Design review of the part shown in the three views and the two pictorial views. Dimensions are in mm from the part's minimum x, y and z. A direction names the side the tool comes from. Round coordinates to 2 decimals unless told otherwise and drop trailing zeros. Loops run counter-clockwise (first coordinate to the right, second up) from the corner with the lowest first, then second, coordinate; pieces in that order, holes last.
1) Take a section at B-B (y = 37.5). State the section outline as (x, z) points (3 decimals), then the cut area to 3 significant figures.
2) Take a section at D-D (y = 10.5). State the section outline as (x, z) points, then the cut area to 3 significant figures.
3) Insertion check: pin 1 (7.5 mm diameter, centred on x = 4, z = 17, fed in from -Y); pin 2 (4.5 mm diameter, centred on x = 7.5, y = 37.5, fed in from -Z); pin 3 (7.5 mm diameter, centred on x = 4.5, z = 15, fed in from +Y); pin 4 (2 mm diameter, centred on y = 16.5, z = 5, fed in from +X). Each pin has a flat end and moves straight along its axis. Give the tip position at first contact, or say it passes through.
4) Wall thickness on L1, parallel to X at y = 37.5, z = 37.95 (3 decimals); L2, parallel to Y at x = 10.25, z = 26; L3, parallel to Z at x = 9.75, y = 38: over which ranges is each line inside the solid? List them lowest first.
5) Take a section at C-C (z = 27.5). State the section outline as (x, y) points, then the cut area to 3 significant figures.
6) Take a section at A-A (x = 7.5). State the section outline as (y, z) points (3 decimals), then the cut area to 3 significant figures.
7) Tool access review of the marked faces 1, 2, 3 and 4: name each direction out of +Z, -Z, +X, -X, +Y, -Y from which nothing blocks a thin tool from reaching the whole face with its end or side.
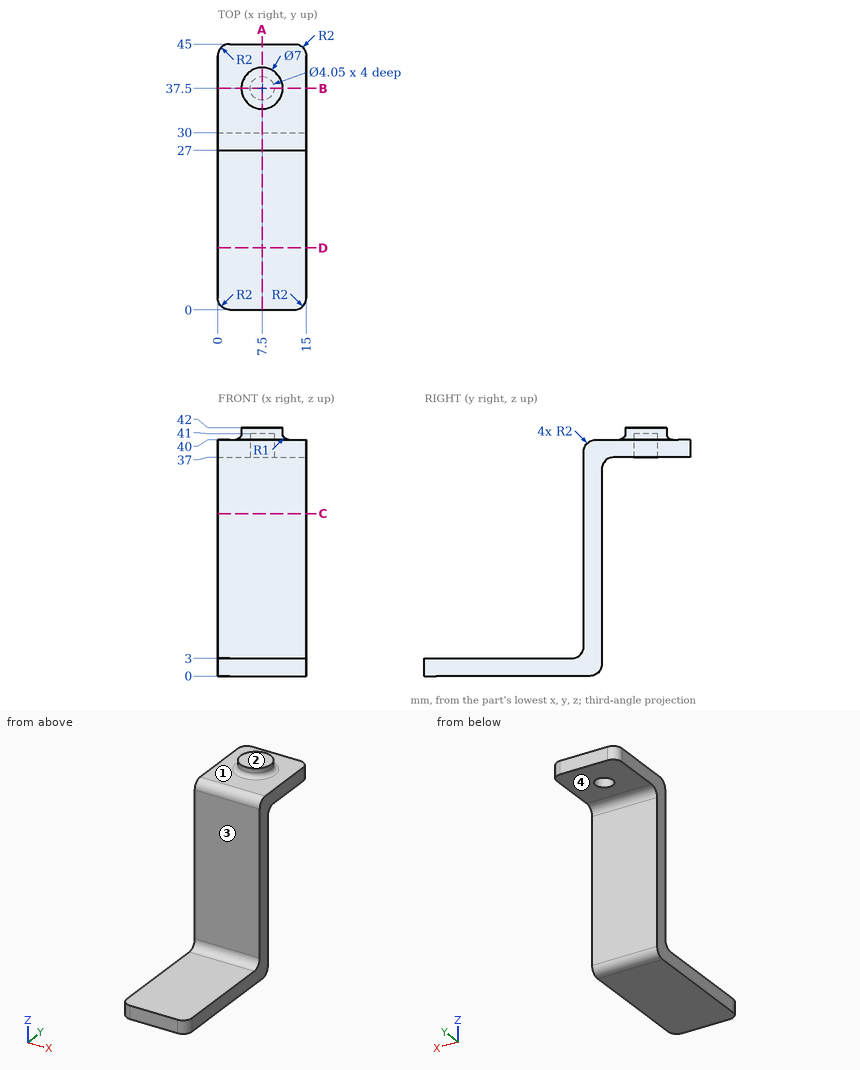
Response:
1. outline: (0, 37) - (5.475, 37) - (5.475, 41) - (9.525, 41) - (9.525, 37) - (15, 37) - (15, 40) - (12, 40) arc R1 cw to (11, 41) - (11, 42) - (4, 42) - (4, 41) arc R1 cw to (3, 40) - (0, 40) - close
1. area: 43.2 mm2
2. outline: (0, 0) - (15, 0) - (15, 3) - (0, 3) - close
2. area: 45.0 mm2
3. pin 1: stops at y = 27
3. pin 2: stops at z = 37
3. pin 3: stops at y = 30
3. pin 4: passes through
4. L1: x = 0 to 5.475, 9.525 to 15
4. L2: y = 27 to 30
4. L3: z = 37 to 42
5. outline: (0, 27) - (15, 27) - (15, 30) - (0, 30) - close
5. area: 45.0 mm2
6. outline: (0, 0) - (28, 0) arc R2 ccw to (30, 2) - (30, 35) arc R2 cw to (32, 37) - (35.475, 37) - (35.475, 41) - (39.525, 41) - (39.525, 37) - (45, 37) - (45, 40) - (42, 40) arc R1 cw to (41, 41) - (41, 42) - (34, 42) - (34, 41) arc R1 cw to (33, 40) - (29, 40) arc R2 ccw to (27, 38) - (27, 5) arc R2 cw to (25, 3) - (0, 3) - close
6. area: 244 mm2
7. face 1: +Z
7. face 2: +Z, +X, -X, +Y, -Y
7. face 3: +Z, +X, -X, -Y
7. face 4: -Z, +X, -X, +Y
